Work out the finished part from the listing and answer in its coordinate system (mm). A direction names the side the tool comes from. Give positions to 0.01 mm unless a question says otherwise; leave off trailing zeros. Loops run counter-clockwise (first coordinate to the right, second up) from the corner with the lowest first, then second, coordinate; pieces in that order, holes last. Notation, with made-up numbers: (-8.75, 70.5) - (9.25, 70.5) arc R14 ccw to (9.25, 93.5) - close; hole circle Ø4 at (-30.75, -40). An arc over 180 degrees is marked (long way). One line per item, written item: value.
from build123d import *

# Parameters (mm, degrees)
BOSS_EXTRU_1_DEPTH      = 50
ESQUISSE2_R             = 1.25
ENL_V_MAT_EXTRU_1_DEPTH = 37.5
ESQUISSE3_R             = 1.5
ENL_V_MAT_EXTRU_2_DEPTH = 13.5


with BuildPart() as part:
    # Esquisse1 → Boss.-Extru.1 (new body)
    with BuildSketch(Plane(origin=(0, 0, 0), x_dir=(1, 0, 0), z_dir=(0, 1, 0))):
        Polygon((0, 0), (35, 0), (35, 7.5), (7.5, 7.5), (7.5, 52.5), (0, 52.5), align=None)
    extrude(amount=BOSS_EXTRU_1_DEPTH)

    # Esquisse2 → Enlèv. mat.-Extru.1 (cut)
    with BuildSketch(Plane.XY):
        with Locations((22.5, 30)):
            Circle(ESQUISSE2_R)
        with Locations((22.5, 20)):
            Circle(ESQUISSE2_R)
        with Locations((12.5, 20)):
            Circle(ESQUISSE2_R)
        with Locations((12.5, 30)):
            Circle(ESQUISSE2_R)
    extrude(amount=-ENL_V_MAT_EXTRU_1_DEPTH, mode=Mode.SUBTRACT)

    # Esquisse3 → Enlèv. mat.-Extru.2 (cut)
    with BuildSketch(Plane.ZY.offset(-7.5)):
        with Locations(Location((-30, 5.55, 0), (0, 0, 180))):
            Circle(ESQUISSE3_R)
        with Locations((-46.844194104, 34.725)):
            Circle(ESQUISSE3_R)
        with Locations((-13.155805896, 34.725)):
            Circle(ESQUISSE3_R)
    extrude(amount=ENL_V_MAT_EXTRU_2_DEPTH, mode=Mode.SUBTRACT)


solid = part.part
1. For faces 4 (the cylindrical face through (23.655, 29.521, -3.698)), 5 (the flat face through (7.5, 25, -30)), determine the directions among +Z, -Z, +X, -X, +Y, -Y from which every point of the face is accessible in a straight line to the end or side of a thin tool.
Output:
face 4: +Z, -Z
face 5: -Z, +X, +Y, -Y
2. Find the intervals of material crossed by line 1 along Y through (x, z) = (22.5, -4.5); line 2 along Z through (x, y) = (2, 5.55); line 3 along Z through (x, y) = (23.5, 10), in increasing order.
Output:
line 1: y = 0 to 18.75, 21.25 to 28.75, 31.25 to 50
line 2: z = -52.5 to -31.5, -28.5 to 0
line 3: z = -7.5 to 0
3. Section A-A (x = 12.5) is taken. Write down the section's boundary in (y, z).
Output:
outline: (0, -7.5) - (18.75, -7.5) - (18.75, 0) - (0, 0) - close; (21.25, -7.5) - (28.75, -7.5) - (28.75, 0) - (21.25, 0) - close; (31.25, -7.5) - (50, -7.5) - (50, 0) - (31.25, 0) - close
4. The mould has two halves that part along Y. Classify faces 1 (the cylindrical face through (3.8, 5.5, -28.5)), 2 (the flat face through (7, 50, -21)), 3 (the flat face through (0, 25, -27)): released by +Y, released by -Y, zero draft, split by the parting line, or undercut.
Output:
face 1: undercut
face 2: released by +Y
face 3: zero draft
5. Section D-D (y = 42) is taken. Write down the section's boundary in (x, z).
Output:
outline: (0, -52.5) - (7.5, -52.5) - (7.5, -7.5) - (35, -7.5) - (35, 0) - (0, 0) - close
6. Flat-ended cylindrical pins translate along their axes: pin 1 Ø14 at (x, y) = (19.5, 14) entering from -Z; pin 2 Ø6 at (y, z) = (42.5, -32) entering from +X. Find the tip coordinate at first contact, or state that the pin passes through.
Output:
pin 1: stops at z = -7.5
pin 2: stops at x = 7.5
7. Section B-B (y = 20) is taken. Write down the section's boundary in (x, z).
Output:
outline: (0, -52.5) - (7.5, -52.5) - (7.5, -7.5) - (11.25, -7.5) - (11.25, 0) - (0, 0) - close; (13.75, -7.5) - (21.25, -7.5) - (21.25, 0) - (13.75, 0) - close; (23.75, -7.5) - (35, -7.5) - (35, 0) - (23.75, 0) - close
8. Section C-C (z = -30) is taken. Write down the section's boundary in (x, y).
Output:
outline: (0, 0) - (7.5, 0) - (7.5, 4.05) - (0, 4.05) - close; (0, 7.05) - (7.5, 7.05) - (7.5, 50) - (0, 50) - close
